Work out the finished part from the listing and answer in its coordinate system (mm). Coordinates: 2 decimals unless noted, no trailing zeros. Write each loop counter-clockwise with the first axis right and the second up, starting at its lowest first coordinate (ties: lowest second). Pieces come first, ordered by that corner, then holes. Notation, with made-up numbers: (80, -25) - (137, -25) arc R17 ccw to (137, -11) - close; hole circle Ø6 at (-27, -3.5). An arc over 180 degrees is marked (long way). One line per item, written item: value.
```python
from build123d import *

# Parameters (mm, degrees)
SKETCH1_W                          = 111
SKETCH1_H                          = 86
BASE_DEPTH                         = 4
NEMA_17_SCREW_HOLE_PATTERN_D       = 3.4
SKETCH5_R                          = 12
MOTOR_SHAFT_BOSS_CLEAREANCE_DEPTH  = 141.474196919
WOOD_SCREW_HOLE_PATTERN_AT_2_COUNT = 2
WOOD_SCREW_HOLE_PATTERN_AT_2_PITCH = 115.20850663
WOOD_SCREW_HOLE_PATTERN_AT_3_COUNT = 2
WOOD_SCREW_HOLE_PATTERN_AT_3_PITCH = 68
WOOD_SCREW_HOLE_PATTERN_AT_4_COUNT = 2
WOOD_SCREW_HOLE_PATTERN_AT_4_PITCH = 93


with BuildPart() as part:
    # Sketch1 → base (new body)
    with BuildSketch(Plane.XY):
        with Locations((55.5, 43)):
            Rectangle(SKETCH1_W, SKETCH1_H)
    extrude(amount=BASE_DEPTH)

    # nema 17 screw hole pattern (through all)
    with Locations(Plane.XY.offset(4)):
        with Locations((40, 58.5), (71, 27.5), (40, 27.5), (71, 58.5)):
            Hole(NEMA_17_SCREW_HOLE_PATTERN_D / 2)

    # Sketch5 → motor shaft boss cleareance (cut, through all)
    with BuildSketch(Plane.XY.offset(4)):
        with Locations((55.5, 43)):
            Circle(SKETCH5_R)
    extrude(amount=-MOTOR_SHAFT_BOSS_CLEAREANCE_DEPTH, mode=Mode.SUBTRACT)

    # Sketch7 → wood screw hole pattern (revolve, cut)
    with BuildSketch(Plane(origin=(9, 77, 4), x_dir=(0, -1, 0), z_dir=(1, 0, 0))):
        Polygon((0, 0), (0, 4), (2.5527, 4), (2.5527, 1.960808018), (4.8895, 0), align=None)
    wood_screw_hole_pattern = revolve(axis=Axis((9, 77, 10.35), (0, 0, -1)), mode=Mode.SUBTRACT)

    # wood screw hole pattern at 2: wood screw hole pattern ×2
    with Locations(*[Vector(0.8072320588129593, -0.5902341935406581, 0) * (i * WOOD_SCREW_HOLE_PATTERN_AT_2_PITCH) for i in range(1, WOOD_SCREW_HOLE_PATTERN_AT_2_COUNT)]):
        add(wood_screw_hole_pattern, mode=Mode.SUBTRACT)

    # wood screw hole pattern at 3: wood screw hole pattern ×2
    with Locations(*[(0, -i * WOOD_SCREW_HOLE_PATTERN_AT_3_PITCH, 0) for i in range(1, WOOD_SCREW_HOLE_PATTERN_AT_3_COUNT)]):
        add(wood_screw_hole_pattern, mode=Mode.SUBTRACT)

    # wood screw hole pattern at 4: wood screw hole pattern ×2
    with Locations(*[(i * WOOD_SCREW_HOLE_PATTERN_AT_4_PITCH, 0, 0) for i in range(1, WOOD_SCREW_HOLE_PATTERN_AT_4_COUNT)]):
        add(wood_screw_hole_pattern, mode=Mode.SUBTRACT)


solid = part.part
```
Item 1: Section C-C, the plane y = 27.5 is taken. Determine the outline of the cut face in (x, z).
Evaluation:
outline: (0, 0) - (38.3, 0) - (38.3, 4) - (0, 4) - close; (41.7, 0) - (69.3, 0) - (69.3, 4) - (41.7, 4) - close; (72.7, 0) - (111, 0) - (111, 4) - (72.7, 4) - close
Item 2: Determine the mould class of faces 1 (the face through (41.25, 59.65, 1.97)), 2 (the face through (42, 44, 4)), 3 (the face through (55, 0, 2)), 4 (the face through (55, 86, 2)) for opening direction Y: +Y half, -Y half, draft (parallel to the pull), parting line (faces both ways), or undercut.
Evaluation:
face 1: undercut
face 2: draft
face 3: -Y half
face 4: +Y half
Item 3: Section D-D, the plane z = 0.7 is taken. Give the number of separate pieces and of enclosed holes in the cut face, then the cut area to 3 significant figures.
Evaluation:
separate pieces: 1
enclosed holes: 9
area: 8,980 mm2
Item 4: Consider probe 1 along X at (y, z) = (77, 0.4); probe 2 along Y at (x, z) = (40, 0.8); probe 3 along Y at (x, z) = (102, 0.95). Determine where each line is inside the solid, lowest interval first.
Evaluation:
probe 1: x = 0 to 6.45, 11.55 to 99.45, 104.55 to 111
probe 2: y = 0 to 25.8, 29.2 to 56.8, 60.2 to 86
probe 3: y = 0 to 6.45, 11.55 to 74.45, 79.55 to 86
Item 5: Section B-B, the plane x = 9 is taken. Determine the outline of the cut face in (y, z), then the cut area to 3 significant figures.
Evaluation:
outline: (0, 0) - (6.45, 0) - (6.45, 2.04) - (4.11, 4) - (0, 4) - close; (11.55, 0) - (74.45, 0) - (74.45, 2.04) - (72.11, 4) - (13.89, 4) - (11.55, 2.04) - close; (79.55, 0) - (86, 0) - (86, 4) - (81.89, 4) - (79.55, 2.04) - close
area: 294 mm2
Item 6: Section A-A, the plane y = 43 is taken. Determine the outline of the cut face in (x, z), then the cut area to 3 significant figures.
Evaluation:
outline: (0, 0) - (43.5, 0) - (43.5, 4) - (0, 4) - close; (67.5, 0) - (111, 0) - (111, 4) - (67.5, 4) - close
area: 348 mm2
